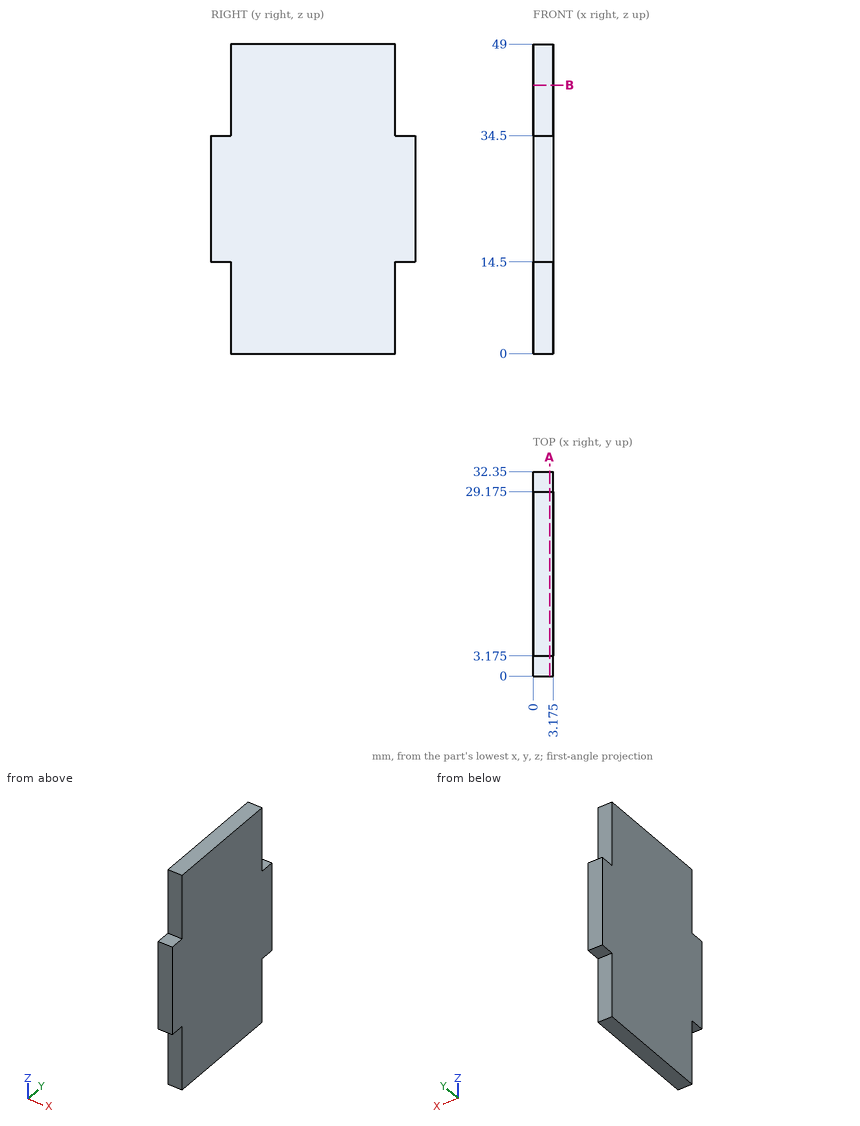
The drawing under review shows one solid part. Ordinate dimensions are in mm from its lowest x, y, z. Round coordinates to 2 decimals unless told otherwise and drop trailing zeros. Write each loop counter-clockwise with the first axis right and the second up, starting at its lowest first coordinate (ties: lowest second). Pieces come first, ordered by that corner, then holes. Notation, with made-up numbers: (1.25, -28.75) - (25.25, -28.75) arc R24 ccw to (25.25, -2.75) - close; hole circle Ø6 at (28, 78). An arc over 180 degrees is marked (long way). Use a Markdown table: item, result. Add a question column.
1. We need section B-B (z = 42.5). State the section outline as (x, y) points (3 decimals), then the cut area to 4 significant figures.
2. Clearance check with flat-ended pins moving along their axes: pin 1 (1.6 mm diameter, centred on x = 1, y = 2, fed in from +Z); pin 2 (1.6 mm diameter, centred on x = 1.5, y = 1, fed in from -Z); pin 3 (1.6 mm diameter, centred on x = 1.5, z = 7.5, fed in from +Y) (3 decimals). State where each tip first meets the part, or that it passes through.
3. Wall thickness on probe 1 along Z at (x, y) = (0.4, 2); probe 2 along Y at (x, z) = (2.95, 10) (3 decimals): over which ranges is each line inside the solid? List them lowest first.
4. We need section A-A (x = 2.6). State the section outline as (y, z) points (3 decimals).
Output:
| question | item | result |
|---|---|---|
| 1 | outline | (0, 3.175) - (3.175, 3.175) - (3.175, 29.175) - (0, 29.175) - close |
| 1 | area | 82.55 mm2 |
| 2 | pin 1 | stops at z = 34.5 |
| 2 | pin 2 | stops at z = 14.5 |
| 2 | pin 3 | stops at y = 29.175 |
| 3 | probe 1 | z = 14.5 to 34.5 |
| 3 | probe 2 | y = 3.175 to 29.175 |
| 4 | outline | (0, 14.5) - (3.175, 14.5) - (3.175, 0) - (29.175, 0) - (29.175, 14.5) - (32.35, 14.5) - (32.35, 34.5) - (29.175, 34.5) - (29.175, 49) - (3.175, 49) - (3.175, 34.5) - (0, 34.5) - close |
